Source: three-view drawing plus pictorial views. Frame: mm from the lowest corner of the part. A direction names the side the tool comes from. Round coordinates to 2 decimals unless told otherwise and drop trailing zeros. Write each loop counter-clockwise with the first axis right and the second up, starting at its lowest first coordinate (ties: lowest second). Pieces come first, ordered by that corner, then holes. Notation, with made-up numbers: M 13.5,-18.75 L 62.5,-18.75 A16 cw 62.5,10.25 Z; hole C 42,78 d7. An arc over 180 degrees is marked long. Put each result on its own line as item: value. Start each with the question number.
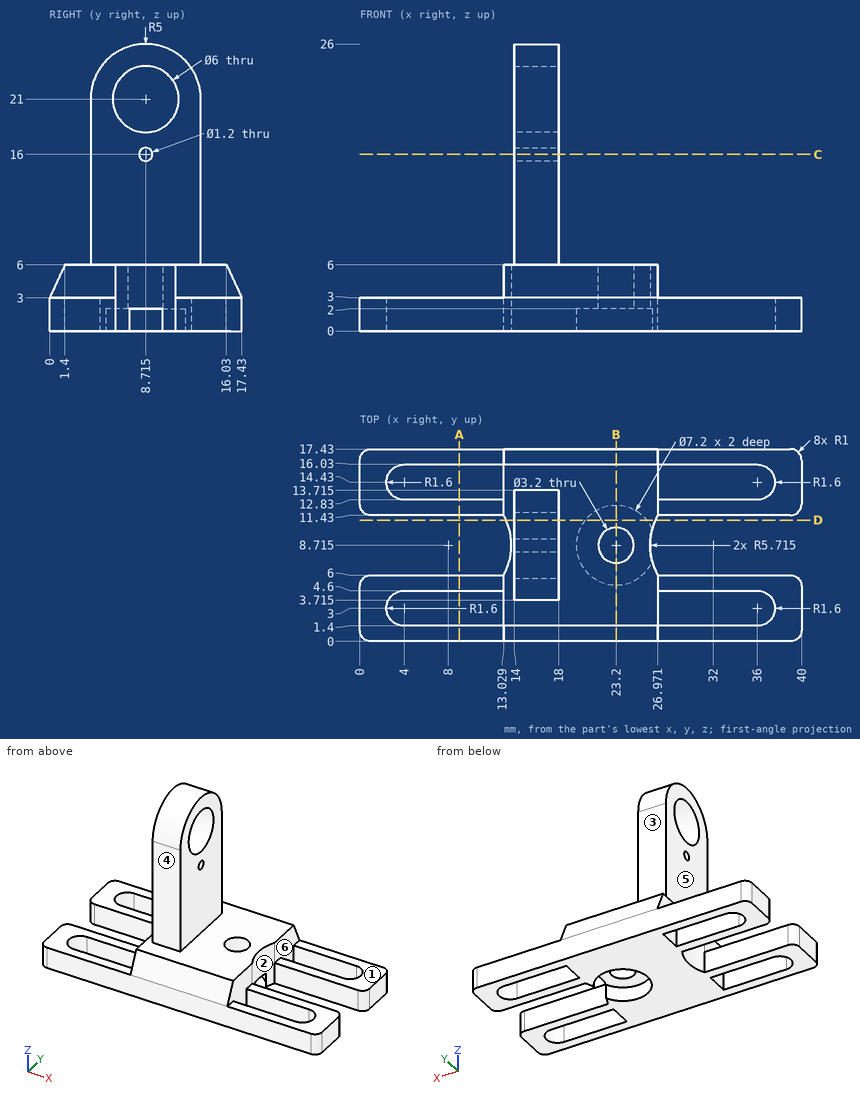
(1) Section query D-D (y = 11). Return loops of the section in (x, z), and give its area (3 significant figures).
(2) Contact query for flat-ended pins moving along their axis: P1, Ø5, axis at x = 31, y = 8, coming from the +Z side; P2, Ø8, axis at y = 11, z = 14.5, coming from the -X side; P3, Ø1.4, axis at y = 8.715, z = 16, coming from the +X side. Output: stop coordinate, or through.
(3) Section query B-B (x = 23.2). Return loops of the section in (y, z) (3 decimals).
(4) Access query for the marked faces 4, 5 and 6. Directions: +Z, -Z, +X, -X, +Y, -Y. A direction counts if a zero-diameter tool reaches every point of the face in a straight line with its end or side. Return the directions, or none.
(5) Section query C-C (z = 16). Return loops of the section in (x, y) (3 decimals).
(6) Section query A-A (x = 9). Return loops of the section in (y, z).
(7) Ray query, line 1 along Y through (x, z) = (15.15, 16) (3 decimals); line 2 along Y through (x, z) = (11.5, 2.75); line 3 along Y through (x, z) = (23.2, 1.05) (3 decimals). Return the intervals inside material, ascending.
(8) Pull-direction query (Y, two-part tool) for the marked faces 1, 2 and 3; classes: +Y half, -Y half, draft (parallel to the pull), parting line (faces both ways), or undercut.
Entries:
1. outline: M 13.24,0 L 20.42,0 L 20.42,2 L 25.98,2 L 25.98,0 L 26.76,0 L 26.76,6 L 18,6 L 18,19.06 L 14,19.06 L 14,6 L 13.24,6 Z; M 14,22.94 L 18,22.94 L 18,25.45 L 14,25.45 Z
1. area: 132 mm2
2. P1: z = 3
2. P2: x = 14
2. P3: x = 18
3. outline: M 0,0 L 5.115,0 L 5.115,2 L 7.115,2 L 7.115,6 L 1.4,6 L 0,3 Z; M 10.315,2 L 12.315,2 L 12.315,0 L 17.43,0 L 17.43,3 L 16.03,6 L 10.315,6 Z
4. face 4: +Z, +X, -X, -Y
4. face 5: +Z, -X, +Y, -Y
4. face 6: +Z
5. outline: M 14,3.715 L 18,3.715 L 18,8.115 L 14,8.115 Z; M 14,9.315 L 18,9.315 L 18,13.715 L 14,13.715 Z
6. outline: M 0,0 L 1.4,0 L 1.4,3 L 0,3 Z; M 4.6,0 L 6,0 L 6,3 L 4.6,3 Z; M 11.43,0 L 12.83,0 L 12.83,3 L 11.43,3 Z; M 16.03,0 L 17.43,0 L 17.43,3 L 16.03,3 Z
7. line 1: 3.715 to 8.115, 9.315 to 13.715
7. line 2: 0 to 1.4, 4.6 to 6, 11.43 to 12.83, 16.03 to 17.43
7. line 3: 0 to 5.115, 12.315 to 17.43
8. face 1: draft
8. face 2: undercut
8. face 3: +Y half
